Geometry check sheet. Reference: drawing and pictorial views, mm from the part's lowest x, y, z. A direction names the side the tool comes from. Round coordinates to 2 decimals unless told otherwise and drop trailing zeros. Order: outer loops, then holes, each group sorted by start corner. A loop starts at its lowest first (then second) coordinate and runs counter-clockwise, first axis right, second up.
(1) Thickness scan on L1, parallel to X at y = 16.8, z = 18; L2, parallel to X at y = 1.5, z = 4.5; L3, parallel to X at y = 18.75, z = 5.5. Record the ranges inside material, lowest first.
(2) Gauge pin test, flat ends, axial feed: P1, Ø5, axis at y = 11.5, z = 11, coming from the -X side; P2, Ø12, axis at x = 94, z = 23.5, coming from the -Y side; P3, Ø5, axis at x = 221, z = 18.5, coming from the -Y side; P4, Ø10, axis at x = 73.5, z = 5.5, coming from the +Y side. Record the tip position at first contact, or that the pin passes through.
(3) Cross-section at A-A on x = 148. Enter the section's corners in (y, z).
(4) Cross-section at B-B on z = 11. Enter the section's corners in (x, y), and give its area (3 significant figures).
(5) Set-up check for the marked faces 4 and 5: record each of +Z, -Z, +X, -X, +Y, -Y from which the full face is reachable in a straight line by a thin tool's end or side.
(6) Draft check along X on the marked faces 1, 2 and 3. Enter one of: pulls with the +X half, pulls with the -X half, needs draft (parallel to the pull), parting line crosses it, or undercut.
(7) Cross-section at D-D on x = 221. Enter the section's corners in (y, z).
(8) Cross-section at C-C on y = 5.5. Enter the section's corners in (x, z), and give its area (3 significant figures).
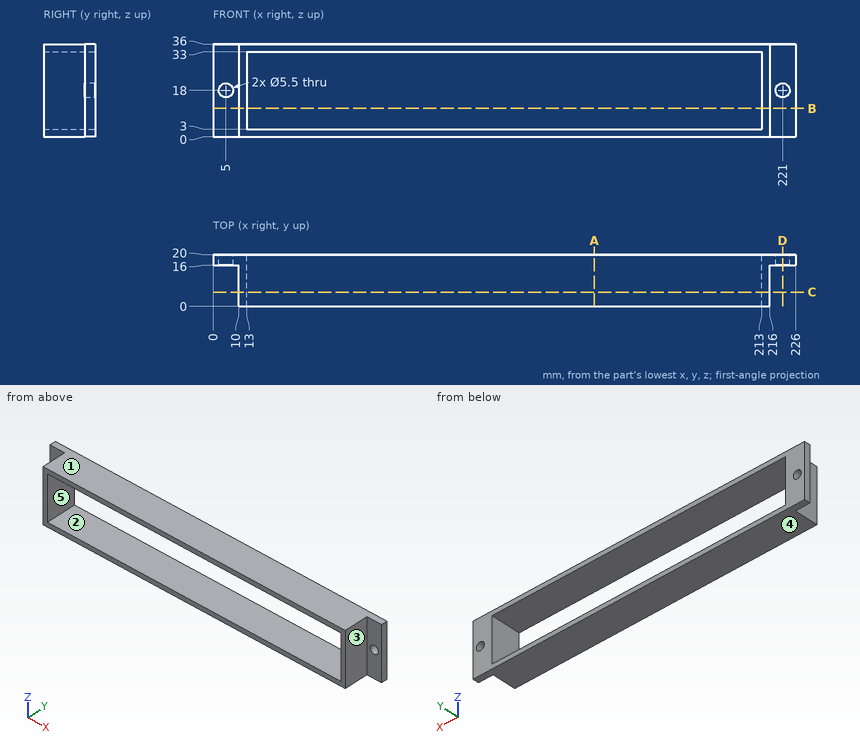
Found:
1. L1: x = 0 to 2.25, 7.75 to 13, 213 to 218.25, 223.75 to 226
1. L2: x = 10 to 13, 213 to 216
1. L3: x = 0 to 13, 213 to 226
2. P1: stops at x = 10
2. P2: passes through
2. P3: stops at y = 16
2. P4: stops at y = 20
3. outline: (0, 0) - (20, 0) - (20, 3) - (0, 3) - close; (0, 33) - (20, 33) - (20, 36) - (0, 36) - close
4. outline: (0, 16) - (10, 16) - (10, 0) - (13, 0) - (13, 20) - (0, 20) - close; (213, 0) - (216, 0) - (216, 16) - (226, 16) - (226, 20) - (213, 20) - close
4. area: 200 mm2
5. face 4: -Z, +X, -X, +Y, -Y
5. face 5: +Y, -Y
6. face 1: needs draft
6. face 2: undercut
6. face 3: pulls with the +X half
7. outline: (16, 0) - (20, 0) - (20, 15.25) - (16, 15.25) - close; (16, 20.75) - (20, 20.75) - (20, 36) - (16, 36) - close
8. outline: (10, 0) - (216, 0) - (216, 36) - (10, 36) - close; hole (13, 3) - (213, 3) - (213, 33) - (13, 33) - close
8. area: 1,420 mm2
